Source: CAD feature listing. Evaluate the final solid. Frame: model axes, mm. Face numbers are marked on the shaded views. A direction names the side the tool comes from. Coordinates: 2 decimals unless noted, no trailing zeros. Write each loop counter-clockwise with the first axis right and the second up, starting at its lowest first coordinate (ties: lowest second). Pieces come first, ordered by that corner, then holes. Notation, with made-up numbers: M 9.5,27 L 29.5,27 A8 cw 29.5,36 Z; hole C 87,-32.75 d3. An arc over 180 degrees is marked long. Write item = value, one per line. Start each with the question number.
1. Section query C-C (y = 0.5). Output: boundary loops of the cut face in (x, z).
2. Pin query (flat end, axial travel): pin 1 Ø3 at (x, y) = (12, 0) entering from -Z; pin 2 Ø0.5 at (y, z) = (-7.5, 6) entering from +X; pin 3 Ø4 at (x, z) = (-9.5, 3.5) entering from +Y; pin 4 Ø0.8 at (x, z) = (11.5, 4) entering from -Y. Return the tip coordinate at first contact, or that it passes through.
3. Section query B-B (x = -3.5). Output: boundary loops of the cut face in (y, z).
4. Pull-direction query (X, two-part tool) for the marked faces 1, 2, 3 and 4; classes: pulls with the +X half, pulls with the -X half, needs draft (parallel to the pull), parting line crosses it, or undercut.
5. Section query D-D (z = 4.5). Give the number of separate pieces and of enclosed holes in the cut face, then the cut area to 3 significant figures.
6. Section query A-A (z = 6.5). Output: boundary loops of the cut face in (x, y), then the cut area to 3 significant figures.
7. Access query for the marked faces 5, 6 and 7. Directions: +Z, -Z, +X, -X, +Y, -Y. A direction counts if a zero-diameter tool reaches every point of the face in a straight line with its end or side. Return the directions, or none.
8. Line query: line 1 along Y through (x, z) = (-3.5, 1.5); line 2 along Y through (x, z) = (0, 3.5); line 3 along X through (y, z) = (-3.75, 2.75). Output: solid intervals per line, ascending.
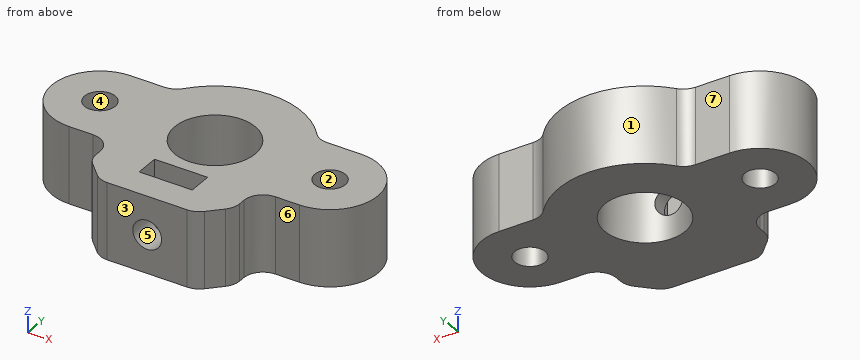
```python
from build123d import *

# Parameters (mm, degrees)
CYLINDER001_R          = 1.5
CYLINDER001_DEPTH      = 15
CYLINDER001_ROLL_ANGLE = 90
PAD002_DEPTH           = 2.5
SKETCH001_R            = 1.6
SKETCH001_R_2          = 4.2
PAD001_DEPTH           = 8
CHAMFER001_SIZE        = 2.5
FILLET001_R            = 2


with BuildPart() as cylinder001:
    # Cylinder001 → Cylinder001 (new body)
    with BuildSketch(Plane.XY):
        Circle(CYLINDER001_R)
    extrude(amount=CYLINDER001_DEPTH)


with BuildPart() as cylinder001_1:
    # Cylinder001 roll: moved
    add(cylinder001.part.rotate(Axis((0, 0, 0), (1, 0, 0)), CYLINDER001_ROLL_ANGLE))


with BuildPart() as cylinder001_2:
    # Cylinder001 placement: moved
    add(cylinder001_1.part.moved(Location((0, 0, 4))))


with BuildPart() as fusion005:
    # Sketch002 → Pad002 (new body)
    with BuildSketch(Plane.XZ.offset(8)):
        Polygon((0, 0.8), (2.771281, 2.4), (2.771281, 5.6), (2.771281, 11.6), (-2.771281, 11.6), (-2.771281, 5.6), (-2.771281, 2.4), align=None)
    extrude(amount=-PAD002_DEPTH)

    # Fusion005: union Cylinder001
    add(cylinder001_2.part)


with BuildPart() as cut002:
    # Sketch001 → Pad001 (new body)
    with BuildSketch(Plane.XY):
        with BuildLine():
            ThreePointArc((-12.000024, 5), (-17, 0), (-12.000024, -5))
            Line((-7.5, -5), (-12.000024, -5))
            Line((-7.5, -11), (-7.5, -5))
            Line((7.5, -11), (-7.5, -11))
            Line((7.5, -5), (7.5, -11))
            Line((12.000024, -5), (7.5, -5))
            ThreePointArc((12.000024, -5), (17, 0), (12.000024, 5))
            Line((7.483315, 5), (12.000024, 5))
            ThreePointArc((7.483315, 5), (0, 9), (-7.483315, 5))
            Line((-12.000024, 5), (-7.483315, 5))
        make_face()
        with Locations((-12, 0)):
            Circle(SKETCH001_R, mode=Mode.SUBTRACT)
        Circle(SKETCH001_R_2, mode=Mode.SUBTRACT)
        with Locations((12, 0)):
            Circle(SKETCH001_R, mode=Mode.SUBTRACT)
    extrude(amount=PAD001_DEPTH)

    # Chamfer001
    chamfer001_edges = [cut002.edges().sort_by_distance(p)[0] for p in [
        (-7.5, -11, 4),
        (7.5, -11, 4),
    ]]
    chamfer(chamfer001_edges, length=CHAMFER001_SIZE)

    # Fillet001
    fillet001_edges = [cut002.edges().sort_by_distance(p)[0] for p in [
        (-7.5, -8.5, 4),
        (-7.5, -5, 4),
        (-5, -11, 4),
        (5, -11, 4),
        (7.5, -8.5, 4),
        (-7.483315, 5, 4),
        (7.5, -5, 4),
        (7.483315, 5, 4),
    ]]
    fillet(fillet001_edges, radius=FILLET001_R)

    # Cut002: cut Fusion005
    add(fusion005.part, mode=Mode.SUBTRACT)


solid = cut002.part
```
Results are:
q1.outline = M -16.97,0 L -13.52,0 L -13.52,8 L -16.97,8 Z; M -10.48,0 L -4.17,0 L -4.17,8 L -10.48,8 Z; M 4.17,0 L 10.48,0 L 10.48,8 L 4.17,8 Z; M 13.52,0 L 16.97,0 L 16.97,8 L 13.52,8 Z
q2.pin_1 = through
q2.pin_2 = 7.5
q2.pin_3 = 5.26
q2.pin_4 = -5
q3.outline = M -11,0 L -2.32,0 L -2.32,8 L -11,8 Z; M 2.32,0 L 8.29,0 L 8.29,8 L 2.32,8 Z
q4.face_1 = parting line crosses it
q4.face_2 = undercut
q4.face_3 = needs draft
q4.face_4 = undercut
q5.separate_pieces = 1
q5.enclosed_holes = 2
q5.area = 348 mm^2
q6.outline = M -12,-5 L -9.5,-5 A2 cw -7.5,-7 L -7.5,-7.67 A2 ccw -6.91,-9.09 L -5.59,-10.41 A2 ccw -4.17,-11 L 4.17,-11 A2 ccw 5.59,-10.41 L 6.91,-9.09 A2 ccw 7.5,-7.67 L 7.5,-7 A2 cw 9.5,-5 L 12,-5 A5 ccw 12,5 L 8.49,5 A2 cw 6.94,5.73 A9 ccw -6.94,5.73 A2 cw -8.49,5 L -12,5 A5 ccw Z; hole C -12,0 d3.2; hole C 0,0 d8.4; hole M -2.77,-8 L 2.77,-8 L 2.77,-5.5 L -2.77,-5.5 Z; hole C 12,0 d3.2
q6.area = 361 mm^2
q7.face_5 = -Y
q7.face_6 = +Z, -Z, +X, -Y
q7.face_7 = +Z, -Z, -X, +Y
q8.line_1 = -11 to -2.32, 2.32 to 8.29
q8.line_2 = 4.2 to 9
q8.line_3 = -15.31 to -1.89, 1.89 to 15.31
